from build123d import *

# Parameters (mm, degrees)
BOSS_EXTRUDE1_DEPTH = 3
SKETCH2_R           = 6.35
SKETCH2_R_2         = 4.7625
CUT_EXTRUDE1_DEPTH  = 129.5846025


with BuildPart() as part:
    # Sketch1 → Boss-Extrude1 (new body)
    with BuildSketch(Plane(origin=(0, 0, 0), x_dir=(0, 0, -1), z_dir=(1, 0, 0))):
        Polygon((-122, 30), (-77, 30), (-77, 27), (-27, 27), (-27, 30), (27, 30), (27, 27), (77, 27), (77, 30), (122, 30), (122, 10), (125, 10), (125, -10), (122, -10), (122, -30), (77, -30), (77, -27), (27, -27), (27, -30), (-27, -30), (-27, -27), (-77, -27), (-77, -30), (-122, -30), (-122, -10), (-125, -10), (-125, 10), (-122, 10), align=None)
    extrude(amount=BOSS_EXTRUDE1_DEPTH)

    # Sketch2 → Cut-Extrude1 (cut, through all)
    with BuildSketch(Plane(origin=(3, 0, 0), x_dir=(0, 0, -1), z_dir=(1, 0, 0))):
        Circle(SKETCH2_R)
        with Locations((-31.75, 0)):
            Circle(SKETCH2_R)
        with Locations(Location((31.75, 0, 0), (0, 0, 180))):
            Circle(SKETCH2_R)
        with Locations((-84.75, 0)):
            Circle(SKETCH2_R_2)
        with Locations(Location((84.75, 0, 0), (0, 0, 180))):
            Circle(SKETCH2_R_2)
    extrude(amount=-CUT_EXTRUDE1_DEPTH, mode=Mode.SUBTRACT)


solid = part.part
Here's how the part is built. I have some questions about the finished solid (model axes, mm). Round coordinates to 2 decimals unless told otherwise and drop trailing zeros. Order: outer loops, then holes, each group sorted by start corner. A loop starts at its lowest first (then second) coordinate and runs counter-clockwise, first axis right, second up. Notation, with made-up numbers: M 69,53.25 L 113,53.25 A19 ccw 113,86.25 Z; hole C 66,75 d9. An arc over 180 degrees is marked long. Return JSON: item names as keys, results as strings. Group by question number.
1. If we section it at C-C on y = 0: List the corners of the cut face in (x, z) for me, then the cut area to 3 significant figures.
2. Please list where these lines run through material, in increasing order: probe 1 along Y at (x, z) = (1.1, 84.75); probe 2 along Y at (x, z) = (2, 0); probe 3 along Z at (x, y) = (0.1, 5.5).
3. If we section it at B-B on x = 0.85: State how many separate pieces and enclosed holes the cut face has, then the cut area to 3 significant figures.
4. If we mould it in two halves opening along Y, with no side actions, what happens to faces 1 (the face through (1.521, 1.907, 25.693)), 2 (the face through (0, 7, -2))? For each: pulls with the +Y half, pulls with the -Y half, needs draft (parallel to the pull), parting line crosses it, or undercut.
5. If we section it at D-D on z = 0: List the corners of the cut face in (x, y) for me.
6. I'm going to push flat-ended pins straight in: pin 1 Ø1.5 at (x, z) = (2, -57.5) entering from +Y; pin 2 Ø1.5 at (x, y) = (2, -29) entering from -Z; pin 3 Ø0.9 at (x, y) = (1, 29) entering from +Z. Where does each tip first touch, or does it pass through?
7. If we section it at A-A on z = 84.75: List the corners of the cut face in (x, y) for me.
Reply:
{
 "1": {"outline": "M 0,-125 L 3,-125 L 3,-89.51 L 0,-89.51 Z; M 0,-79.99 L 3,-79.99 L 3,-38.1 L 0,-38.1 Z; M 0,-25.4 L 3,-25.4 L 3,-6.35 L 0,-6.35 Z; M 0,6.35 L 3,6.35 L 3,25.4 L 0,25.4 Z; M 0,38.1 L 3,38.1 L 3,79.99 L 0,79.99 Z; M 0,89.51 L 3,89.51 L 3,125 L 0,125 Z", "area": "579 mm^2"},
 "2": {"probe 1": "-30 to -4.76, 4.76 to 30", "probe 2": "-30 to -6.35, 6.35 to 30", "probe 3": "-125 to -34.92, -28.58 to -3.17, 3.17 to 28.58, 34.92 to 125"},
 "3": {"separate pieces": "1", "enclosed holes": "5", "area": "13,600 mm^2"},
 "4": {"face 1": "undercut", "face 2": "needs draft"},
 "5": {"outline": "M 0,-30 L 3,-30 L 3,-6.35 L 0,-6.35 Z; M 0,6.35 L 3,6.35 L 3,30 L 0,30 Z"},
 "6": {"pin 1": "y = 27", "pin 2": "z = -122", "pin 3": "z = 122"},
 "7": {"outline": "M 0,-30 L 3,-30 L 3,-4.76 L 0,-4.76 Z; M 0,4.76 L 3,4.76 L 3,30 L 0,30 Z"}
}
